```python
from build123d import *

# Parameters (mm, degrees)
BOSS_EXTRUDE1_DEPTH = 4
SKETCH2_R           = 3
BOSS_EXTRUDE2_DEPTH = 18
SKETCH6_OUTSIDE_W   = 101.492
SKETCH6_OUTSIDE_H   = 103.04
SKETCH6_OUTSIDE_R   = 5
CUT_EXTRUDE1_DEPTH  = 24.2880513
CUT_EXTRUDE1_DRAFT  = -60
CHAMFER1_SIZE       = 0.5


with BuildPart() as part:
    # Sketch1 → Boss-Extrude1 (new body)
    with BuildSketch(Plane.XY):
        Polygon((0, -5.773502692), (5, -2.886751346), (5, 2.886751346), (0, 5.773502692), (-5, 2.886751346), (-5, -2.886751346), align=None)
    extrude(amount=BOSS_EXTRUDE1_DEPTH)

    # Sketch2 → Boss-Extrude2 (add)
    with BuildSketch(Plane.XY.offset(4)):
        Circle(SKETCH2_R)
    extrude(amount=BOSS_EXTRUDE2_DEPTH)


with BuildPart() as cut_extrude1_tool:
    # Sketch6 outside → Cut-Extrude1 (with draft: the straight prism first)
    with BuildSketch(Plane(origin=(0, 0, 0), x_dir=(-1, 0, 0), z_dir=(0, 0, -1))):
        Rectangle(SKETCH6_OUTSIDE_W, SKETCH6_OUTSIDE_H)
        Circle(SKETCH6_OUTSIDE_R, mode=Mode.SUBTRACT)
    extrude(amount=-CUT_EXTRUDE1_DEPTH)
    # Cut-Extrude1: the draft: its side faces are tilted about the plane it starts from
    cut_extrude1_sides = [cut_extrude1_tool.faces().sort_by_distance(p)[0] for p in [
        (0, -51.52, 12.14402565),
        (-50.746, 0, 12.14402565),
        (0, 51.52, 12.14402565),
        (50.746, 0, 12.14402565),
        (5, 0, 12.14402565),
    ]]
    draft(cut_extrude1_sides, Plane(origin=(0, 0, 0), x_dir=(-1, 0, 0), z_dir=(0, 0, -1)), CUT_EXTRUDE1_DRAFT)


with BuildPart() as part_1:
    add(part.part)

    # Cut-Extrude1: cut by cut_extrude1_tool
    add(cut_extrude1_tool.part, mode=Mode.SUBTRACT)

    # Chamfer1
    chamfer1_edges = [part_1.edges().sort_by_distance(p)[0] for p in [
        (-3, 0, 22),
    ]]
    chamfer(chamfer1_edges, length=CHAMFER1_SIZE)


solid = part_1.part
```
Geometry check sheet. Reference: the model listing, model coordinates, mm. A direction names the side the tool comes from. Give positions to 0.01 mm unless a question says otherwise; leave off trailing zeros. Loops run counter-clockwise (first coordinate to the right, second up) from the corner with the lowest first, then second, coordinate; pieces in that order, holes last. Notation, with made-up numbers: M 64.5,54.5 L 83.5,54.5 A21 cw 83.5,75.5 Z; hole C -25,35.25 d8. An arc over 180 degrees is marked long. Write item = value, one per line.
(1) Gauge pin test, flat end, axial feed: pin 1 Ø3 at (x, z) = (-3.5, 19.5) entering from +Y. Record the tip position at first contact, or that the pin passes through.
Answer below:
pin_1 = 2.24
(2) Material ranges on line 1 (Z direction, x = 4.5, y = 1); line 2 (Z direction, x = -2.5, y = 1); line 3 (Y direction, x = 2, z = 4.25), recorded low to high. Write a range as [from, to].
Answer below:
line_1 = [0, 4]
line_2 = [0, 21.81]
line_3 = [-2.24, 2.24]
(3) Sectioned sample at A-A, the plane z = 15. Record the cut outline in (x, y).
Answer below:
outline = C 0,0 d6
(4) Tool access check on faces 1 (the face through (-3, 0, 13)), 2 (the face through (4.483, 2.603, 0.106)). Record the directions out of +Z, -Z, +X, -X, +Y, -Y that give a thin tool (end or side, any length) a straight path to the whole face; none if there is none.
Answer below:
face_1 = +Z
face_2 = -Z, +X, +Y
